The model under review builds one solid part; all positions refer to its coordinate system, in mm. Face numbers are marked on the shaded views. Round coordinates to 2 decimals unless told otherwise and drop trailing zeros. Write each loop counter-clockwise with the first axis right and the second up, starting at its lowest first coordinate (ties: lowest second). Pieces come first, ordered by that corner, then holes. Notation, with made-up numbers: (71, -28.75) - (122, -28.75) arc R10 ccw to (122, -19.75) - close; hole circle Ø3 at (-37, 71.5). An arc over 180 degrees is marked (long way). Use one line per item in the form item = value.
from build123d import *

# Parameters (mm, degrees)
F0_R     = 38.1
F1_DEPTH = 101.6
F2_T     = -5.08
F3_R     = 7.62
F4_R     = 2.53999
F5_SIZE  = 5.08


# Not quite as in the source:
# - a fillet or chamfer is up to 0.001 mm smaller than in the source, because OpenCascade refuses the exact size


with BuildPart() as f1:
    # F0 (on Top) → F1 (new body)
    with BuildSketch(Plane.XY):
        with Locations((-51.5342205763, 6.2507814728)):
            Circle(F0_R)
    extrude(amount=F1_DEPTH)

    # F2
    f2_openings = [f1.faces().sort_by_distance(p)[0] for p in [
        (-51.534221, 6.250781, 101.6),
    ]]
    offset(amount=F2_T, openings=f2_openings)

    # F3
    f3_edges = [f1.edges().sort_by_distance(p)[0] for p in [
        (-84.554221, 6.250781, 5.08),
    ]]
    fillet(f3_edges, radius=F3_R)

    # F4 (radius 2.54 in the source; OpenCascade refuses exactly that, so slightly less here)
    f4_edges = [f1.edges().sort_by_distance(p)[0] for p in [
        (-84.554221, 6.250781, 101.6),
        (-89.634221, 6.250781, 101.6),
    ]]
    fillet(f4_edges, radius=F4_R)

    # F5
    f5_edges = [f1.edges().sort_by_distance(p)[0] for p in [
        (-89.634221, 6.250781, 0),
    ]]
    chamfer(f5_edges, length=F5_SIZE)


solid = f1.part
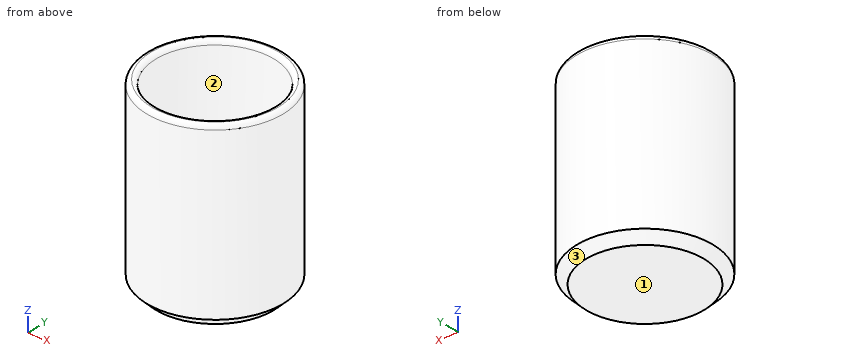
(1) The part is to be moulded in two halves that separate along Y. For the marked faces 1, 2 and 3, say which applies: +Y half, -Y half, draft (parallel to the pull), parting line (faces both ways), or undercut.
Geometry results:
face_1 = draft
face_2 = undercut
face_3 = parting line
(2) Add section A-A on z = 14. Write out the cut boundary in (x, y).
Geometry results:
outline = circle Ø76.2 at (-51.53, 6.25); hole circle Ø66.04 at (-51.53, 6.25)
(3) Insertion check: P1, Ø5, axis at x = -29, z = 18, coming from the -Y side; P2, Ø6, axis at y = 3, z = 54, coming from the -X side; P3, Ø4, axis at y = 34, z = 65.5, coming from the -X side. Each pin has a flat end and moves straight along its axis. Give the tip position at first contact, or say it passes through.
Geometry results:
P1 = -26.16
P2 = -89.63
P3 = -79.62
(4) To check wall thickness, follow L1, parallel to X at y = -0.5, z = 55; L2, parallel to X at y = -14, z = 85; L3, parallel to Y at x = -69.5, z = 11. State the ranges of each line that lie inside material, in increasing order.
Geometry results:
L1 = -89.03 to -83.86, -19.21 to -14.04
L2 = -83.81 to -77.62, -25.45 to -19.26
L3 = -27.35 to -21.22, 33.73 to 39.85
